Build history of the part. All positions in model axes, mm. A direction names the side the tool comes from. Coordinates: 2 decimals unless noted, no trailing zeros. Loops run counter-clockwise (first coordinate to the right, second up) from the corner with the lowest first, then second, coordinate; pieces in that order, holes last.
(1) Wall check: L1, parallel to Z at x = 167.25, y = 33.5; L2, parallel to Y at x = 162.25, z = 297; L3, parallel to X at y = 66.5, z = 296.25. Give the ranges that are in metal, low to high.
(2) Slice it at D-D (x = 166.25). Give the cut face in (y, z), and give its area (3 significant figures).
(3) Two-plate mould, pull along Z, no slides. Class faces 1 (the face through (175, 40, 293.03)), 2 (the face through (175.006, 68.229, 303.122)), 3 (the face through (174.6, 59, 300)): pulls with the +Z half, pulls with the -Z half, needs draft (parallel to the pull), parting line crosses it, or undercut.
(4) Slice it at B-B (z = 304.25). Give the cut face in (x, y).
(5) Slice it at A-A (z = 297.25). Give the cut face in (x, y), and give its area (3 significant figures).
(6) Flat gauge pins, fed straight in: P1, Ø6.5, axis at y = 67.63, z = 305.03, coming from the -X side; P2, Ø6.5, axis at y = 26.5, z = 297.5, coming from the +X side; P3, Ø5, axis at x = 170.5, z = 296, coming from the -Y side. Where does each tip first touch, or does it go through?
(7) Tool access for faces 4 (the face through (168, 34.028, 297)), 5 (the face through (175.4, 59, 300)), 6 (the face through (160.4, 23, 297)): list every direction of +Z, -Z, +X, -X, +Y, -Y with a clear straight run to the whole face (end or side of a thin tool).
(8) Slice it at C-C (y = 21.5). Give the cut face in (x, z), and give its area (3 significant figures).
from build123d import *

# Parameters (mm, degrees)
SKETCH1_W           = 15.8
SKETCH1_H           = 58
BOSS_EXTRUDE1_DEPTH = 8
SKETCH2_W           = 15
SKETCH2_H           = 39.6
CUT_EXTRUDE1_DEPTH  = 191.395014145
SKETCH3_W           = 0.8
SKETCH3_H           = 18.745212198
BOSS_EXTRUDE2_DEPTH = 10
SKETCH4_W           = 15
SKETCH4_H           = 17.6
CUT_EXTRUDE2_DEPTH  = 191.489530975
HOLE1_D             = 4
FILLET1_R           = 2
FILLET2_R           = 2
FILLET3_R           = 2.8
FILLET4_R           = 2.8


with BuildPart() as part:
    # Sketch1 → Boss-Extrude1 (new body)
    with BuildSketch(Plane(origin=(0, 0, 293.029524909), x_dir=(-1, 0, 0), z_dir=(0, 0, -1))):
        with Locations((-167.5, 44.628129211)):
            Rectangle(SKETCH1_W, SKETCH1_H)
    extrude(amount=-BOSS_EXTRUDE1_DEPTH)

    # Sketch2 → Cut-Extrude1 (cut, through all)
    with BuildSketch(Plane(origin=(0, 0, 293.029524909), x_dir=(-1, 0, 0), z_dir=(0, 0, -1))):
        with Locations((-167.1, 53.828129211)):
            Rectangle(SKETCH2_W, SKETCH2_H)
    extrude(amount=-CUT_EXTRUDE1_DEPTH, mode=Mode.SUBTRACT)

    # Sketch3 → Boss-Extrude2 (add)
    with BuildSketch(Plane.XY.offset(301.029524909)):
        with Locations((175, 64.255523112)):
            Rectangle(SKETCH3_W, SKETCH3_H)
    extrude(amount=BOSS_EXTRUDE2_DEPTH)

    # Sketch4 → Cut-Extrude2 (cut, through all)
    with BuildSketch(Plane.XY.offset(301.029524909)):
        with Locations((167.9, 24.428129211)):
            Rectangle(SKETCH4_W, SKETCH4_H)
    extrude(amount=-CUT_EXTRUDE2_DEPTH, mode=Mode.SUBTRACT)

    # Hole1 (through all)
    with Locations(Plane.ZY.offset(-174.6)):
        with Locations((305.029524909, 67.628129211)):
            Hole(HOLE1_D / 2)

    # Fillet1
    fillet1_edges = [part.edges().sort_by_distance(p)[0] for p in [
        (160.4, 33.228129211, 297.029524909),
    ]]
    fillet(fillet1_edges, radius=FILLET1_R)

    # Fillet2
    fillet2_edges = [part.edges().sort_by_distance(p)[0] for p in [
        (174.6, 34.028129211, 297.029524909),
    ]]
    fillet(fillet2_edges, radius=FILLET2_R)

    # Fillet3
    fillet3_edges = [part.edges().sort_by_distance(p)[0] for p in [
        (159.6, 34.028129211, 297.029524909),
    ]]
    fillet(fillet3_edges, radius=FILLET3_R)

    # Fillet4
    fillet4_edges = [part.edges().sort_by_distance(p)[0] for p in [
        (175.4, 33.228129211, 297.029524909),
    ]]
    fillet(fillet4_edges, radius=FILLET4_R)


solid = part.part
Response values:
1. L1: z = 293.03 to 301.03
1. L2: y = 33.22 to 34.02
1. L3: x = 174.6 to 175.4
2. outline: (33.23, 293.03) - (34.03, 293.03) - (34.03, 301.03) - (33.23, 301.03) - close
2. area: 6.40 mm2
3. face 1: pulls with the -Z half
3. face 2: undercut
3. face 3: needs draft
4. outline: (174.6, 54.88) - (175.4, 54.88) - (175.4, 65.79) - (174.6, 65.79) - close; (174.6, 69.47) - (175.4, 69.47) - (175.4, 73.63) - (174.6, 73.63) - close
5. outline: (159.6, 15.63) - (160.4, 15.63) - (160.4, 31.23) arc R2 cw to (162.4, 33.23) - (172.6, 33.23) arc R2.8 ccw to (175.4, 36.03) - (175.4, 73.63) - (174.6, 73.63) - (174.6, 36.03) arc R2 cw to (172.6, 34.03) - (162.4, 34.03) arc R2.8 ccw to (159.6, 31.23) - close
5. area: 56.8 mm2
6. P1: stops at x = 174.6
6. P2: stops at x = 160.4
6. P3: stops at y = 33.23
7. face 4: +Z, -Z, -X, +Y
7. face 5: +Z, -Z, +X, +Y, -Y
7. face 6: +Z, -Z, +X, -Y
8. outline: (159.6, 293.03) - (160.4, 293.03) - (160.4, 301.03) - (159.6, 301.03) - close
8. area: 6.40 mm2
